Verification items for the finished model (mm, model axes). A direction names the side the tool comes from. Coordinates: 2 decimals unless noted, no trailing zeros. Order: outer loops, then holes, each group sorted by start corner. A loop starts at its lowest first (then second) coordinate and runs counter-clockwise, first axis right, second up. Notation, with made-up numbers: M -19,79 L 15,79 A28 cw 15,107 Z; hole C 86,32.25 d11. An arc over 180 degrees is marked long. Write item = value, one per line.
```python
from build123d import *

# Parameters (mm, degrees)
F0_R     = 10
F1_DEPTH = 25
F2_DEPTH = 50
F3_SIZE  = 2


# Not quite as in the source:
# - the program builds the solid bodies; features that only make, move or delete a surface that nothing else refers to are left out


with BuildPart() as f1:
    # F0 (on Front) → F1 (new body)
    with BuildSketch(Plane.XZ):
        with BuildLine():
            ThreePointArc((2.0833333333, -24.9130432148), (18.3995018048, -16.9250800097), (25, 0))
            ThreePointArc((25, 0), (18.3995018048, 16.9250800097), (2.0833333333, 24.9130432148))
            ThreePointArc((2.0833333333, 24.9130432148), (-25, 0), (2.0833333333, -24.9130432148))
        make_face()
        Circle(F0_R, mode=Mode.SUBTRACT)
        with BuildLine():
            ThreePointArc((2.0833333333, 24.9130432148), (18.3995018048, 16.9250800097), (25, 0))
            ThreePointArc((25, 0), (18.3995018048, -16.9250800097), (2.0833333333, -24.9130432148))
            Line((2.0833333333, -24.9130432148), (91.4583333333, -17.4391302504))
            ThreePointArc((91.4583333333, -17.4391302504), (72.5, 0), (91.4583333333, 17.4391302504))
            Line((91.4583333333, 17.4391302504), (2.0833333333, 24.9130432148))
        make_face()
        with BuildLine():
            ThreePointArc((107.5, 0), (102.8796512634, 11.8475560068), (91.4583333333, 17.4391302504))
            ThreePointArc((91.4583333333, 17.4391302504), (72.5, 0), (91.4583333333, -17.4391302504))
            ThreePointArc((91.4583333333, -17.4391302504), (102.8796512634, -11.8475560068), (107.5, 0))
        make_face()
        with Locations((90, 0)):
            Circle(F0_R, mode=Mode.SUBTRACT)
    extrude(amount=F1_DEPTH)

    # F0 (on Front) → F2 (join)
    with BuildSketch(Plane.XZ):
        with BuildLine():
            ThreePointArc((2.0833333333, -24.9130432148), (18.3995018048, -16.9250800097), (25, 0))
            ThreePointArc((25, 0), (18.3995018048, 16.9250800097), (2.0833333333, 24.9130432148))
            ThreePointArc((2.0833333333, 24.9130432148), (-25, 0), (2.0833333333, -24.9130432148))
        make_face()
        Circle(F0_R, mode=Mode.SUBTRACT)
    extrude(amount=F2_DEPTH)

    # F3
    f3_edges = [f1.edges().sort_by_distance(p)[0] for p in [
        (-2.083333, -50, 24.913043),
        (-10, -50, 0),
        (80, -25, 0),
    ]]
    chamfer(f3_edges, length=F3_SIZE)


solid = f1.part
```
Item 1: Sectioned sample at C-C, the plane y = -46.5. Enter the section's corners in (x, z), then the cut area to 3 significant figures.
Report:
outline = C 0,0 d50; hole C 0,0 d20
area = 1,650 mm^2
Item 2: Scan lines: L1, parallel to Y at x = 39.5, z = -12; L2, parallel to Z at x = 0, y = -14.5; L3, parallel to Z at x = -1, y = -16. Record each from-to range of solid material in increasing order. Write a range as from..to.
Report:
L1 = -25..0
L2 = -25..-10, 10..25
L3 = -24.98..-9.95, 9.95..24.98
Item 3: Sectioned sample at A-A, the plane x = 0. Enter the section's corners in (y, z), then the cut area to 3 significant figures.
Report:
outline = M -50,-23 L -48,-25 L 0,-25 L 0,-10 L -48,-10 L -50,-12 Z; M -50,12 L -48,10 L 0,10 L 0,25 L -48,25 L -50,23 Z
area = 1,490 mm^2
Item 4: Sectioned sample at B-B, the plane y = -17. Enter the section's corners in (x, z), then the cut area to 3 significant figures.
Report:
outline = M 2.08,-24.91 L 91.46,-17.44 A17.5 ccw 91.46,17.44 L 2.08,24.91 A25 ccw long Z; hole C 0,0 d20; hole C 90,0 d20
area = 4,670 mm^2
Item 5: Gauge pin test, flat ends, axial feed: pin 1 (2 mm diameter, centred on x = 33, y = -15.5, fed in from -Z); pin 2 (1 mm diameter, centred on x = 75, y = -15.5, fed in from +Z); pin 3 (8 mm diameter, centred on x = 3.5, z = 11.5, fed in from +Y); pin 4 (2 mm diameter, centred on x = 82.5, z = 6, fed in from -Y). Record the tip position at first contact, or that the pin passes through.
Report:
pin_1 = -22.41
pin_2 = 18.86
pin_3 = 0
pin_4 = -23.6
Item 6: Tool access check on faces 4 (the flat face through (10, -50, -10)), 5 (the cylindrical face through (-24.77, -29, 3.37)). Record the directions out of +Z, -Z, +X, -X, +Y, -Y that give a thin tool (end or side, any length) a straight path to the whole face; none if there is none.
Report:
face_4 = +Z, -Z, +X, -X, -Y
face_5 = -Y
Item 7: Sectioned sample at D-D, the plane z = -2. Give the number of separate pieces and of enclosed holes in the cut face, then the cut area to 3 significant figures.
Report:
separate_pieces = 3
enclosed_holes = 0
area = 3,070 mm^2
Item 8: Release check for a two-part mould opening along Z. For faces 1 (the flat face through (54, -25, 0)), 2 (the flat face through (47.396, -12.325, 21.124)), 3 (the cylindrical face through (80, -11, 0)) record: pulls with the +Z half, pulls with the -Z half, needs draft (parallel to the pull), parting line crosses it, or undercut.
Report:
face_1 = needs draft
face_2 = pulls with the +Z half
face_3 = undercut
